```python
from build123d import *

# Parameters (mm, degrees)
F0_W     = 60
F0_H     = 30
F1_DEPTH = 30
F2_W     = 44
F2_H     = 30
F3_DEPTH = 6
F4_W     = 44
F4_H     = 24
F5_DEPTH = 6
F6_W     = 44
F6_H     = 24
F7_DEPTH = 6
F8_W     = 44
F8_H     = 18
F9_DEPTH = 6


with BuildPart() as f1:
    # F0 (on Front) → F1 (new body)
    with BuildSketch(Plane.XZ):
        Rectangle(F0_W, F0_H)
    extrude(amount=F1_DEPTH)

    # F2 (on face) → F3 (cut)
    with BuildSketch(Plane.XZ.offset(30)):
        Rectangle(F2_W, F2_H)
    extrude(amount=-F3_DEPTH, mode=Mode.SUBTRACT)

    # F4 (on face) → F5 (cut)
    with BuildSketch(Plane(origin=(0, 0, -15), x_dir=(1, 0, 0), z_dir=(0, 0, -1))):
        with Locations((0, 12)):
            Rectangle(F4_W, F4_H)
    extrude(amount=-F5_DEPTH, mode=Mode.SUBTRACT)

    # F6 (on face) → F7 (cut)
    with BuildSketch(Plane(origin=(0, 0, 0), x_dir=(-1, 0, 0), z_dir=(0, 1, 0))):
        with Locations((0, 3)):
            Rectangle(F6_W, F6_H)
    extrude(amount=-F7_DEPTH, mode=Mode.SUBTRACT)

    # F8 (on face) → F9 (cut)
    with BuildSketch(Plane.XY.offset(15)):
        with Locations((0, -15)):
            Rectangle(F8_W, F8_H)
    extrude(amount=-F9_DEPTH, mode=Mode.SUBTRACT)


solid = f1.part
```
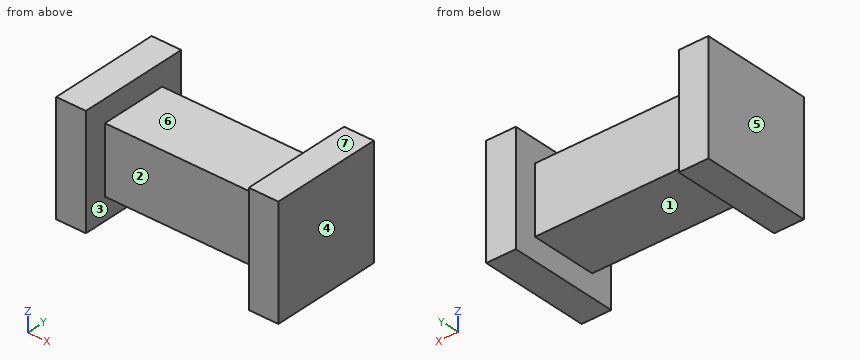
Check sheet for the modelled part. Datum: model origin and axes. Units: mm. Face numbers are marked on the shaded views. A direction names the side the tool comes from. Give positions to 0.01 mm unless a question says otherwise; leave off trailing zeros. Write each loop counter-clockwise with the first axis right and the second up, starting at its lowest first coordinate (ties: lowest second). Pieces come first, ordered by that corner, then holes. Notation, with made-up numbers: (-39, 24) -> (-12, 24) arc R13 ccw to (-12, 30) -> close; hole circle Ø3 at (27.5, -34). An arc over 180 degrees is marked (long way). Use CSV: the item, a comma, the result in double quotes. Start each with the question number.
Q1. Release check for a two-part mould opening along X. For the marked faces 4, 5, 6 and 7 record: +X half, -X half, draft (parallel to the pull), parting line (faces both ways), or undercut.
Q2. Cross-section at A-A on z = -11. Enter the section's corners in (x, y).
Q3. Cross-section at C-C on y = -11. Enter the section's corners in (x, z).
Q4. Cross-section at D-D on z = -2.25. Enter the section's corners in (x, y), and give its area (3 significant figures).
Q5. Depth check by flat-ended pin: P1, Ø1.5, axis at x = 9, z = -6, coming from the +Y side; P2, Ø12, axis at x = -15.5, y = -16, coming from the +Z side; P3, Ø12, axis at x = 5.5, y = -19, coming from the -Z side. Enter the tip coordinate at first touch or a pass-through.
Q6. Scan lines: line 1 along X through (y, z) = (-16.5, 11); line 2 along Y through (x, z) = (15.5, -8); line 3 along Z through (x, y) = (0.5, -22.25). Record each from-to range of solid material in increasing order.
Q7. Tool access check on the marked faces 1, 2 and 3. Record the directions out of +Z, -Z, +X, -X, +Y, -Y that give a thin tool (end or side, any length) a straight path to the whole face; none if there is none.
Q8. Cross-section at B-B on y = -25.75. Enter the section's corners in (x, z).
Working result:
1,face 4,"+X half"
1,face 5,"-X half"
1,face 6,"undercut"
1,face 7,"draft"
2,outline,"(-30, -30) -> (-22, -30) -> (-22, 0) -> (-30, 0) -> close; (22, -30) -> (30, -30) -> (30, 0) -> (22, 0) -> close"
3,outline,"(-30, -15) -> (-22, -15) -> (-22, -9) -> (22, -9) -> (22, -15) -> (30, -15) -> (30, 15) -> (22, 15) -> (22, 9) -> (-22, 9) -> (-22, 15) -> (-30, 15) -> close"
4,outline,"(-30, -30) -> (-22, -30) -> (-22, -24) -> (22, -24) -> (22, -30) -> (30, -30) -> (30, 0) -> (22, 0) -> (22, -6) -> (-22, -6) -> (-22, 0) -> (-30, 0) -> close"
4,area,"1,270 mm^2"
5,P1,"stops at y = -6"
5,P2,"stops at z = 9"
5,P3,"stops at z = -9"
6,line 1,"x = -30 to -22, 22 to 30"
6,line 2,"y = -24 to -6"
6,line 3,"z = -9 to 9"
7,face 1,"-Z, +Y, -Y"
7,face 2,"+Z, -Z, -Y"
7,face 3,"none"
8,outline,"(-30, -15) -> (-22, -15) -> (-22, 15) -> (-30, 15) -> close; (22, -15) -> (30, -15) -> (30, 15) -> (22, 15) -> close"
